The model under review builds one solid part; all positions refer to its coordinate system, in mm. A direction names the side the tool comes from. Coordinates: 2 decimals unless noted, no trailing zeros. Order: outer loops, then holes, each group sorted by start corner. A loop starts at its lowest first (then second) coordinate and runs counter-clockwise, first axis right, second up. Notation, with made-up numbers: (66.25, -37.5) - (104.25, -37.5) arc R15 cw to (104.25, -26.5) - close; hole circle Ø7 at (84.25, 2.25). An arc over 180 degrees is marked (long way). Answer in a Markdown table with one row per item.
```python
from build123d import *

# Parameters (mm, degrees)
SKETCH1_W           = 2
SKETCH1_H           = 16
BOSS_EXTRUDE1_DEPTH = 7.9375
SKETCH1_4_W         = 40
SKETCH1_4_H         = 1
BOSS_EXTRUDE2_DEPTH = 7.9375
LPATTERN1_COUNT     = 6
LPATTERN1_PITCH     = 3


with BuildPart() as part:
    # Sketch1 → Boss-Extrude1 (new body)
    with BuildSketch(Plane(origin=(0, 0, 0), x_dir=(1, 0, 0), z_dir=(0, 1, 0))):
        with Locations((-9.581037754, 12.413793103)):
            Rectangle(SKETCH1_W, SKETCH1_H)
    extrude(amount=BOSS_EXTRUDE1_DEPTH)

    # Sketch1<4> → Boss-Extrude2 (add)
    with BuildSketch(Plane(origin=(0, 0, 0), x_dir=(1, 0, 0), z_dir=(0, 1, 0))):
        with Locations((11.418962246, 19.913793103)):
            Rectangle(SKETCH1_4_W, SKETCH1_4_H)
    boss_extrude2 = extrude(amount=BOSS_EXTRUDE2_DEPTH)

    # LPattern1: Boss-Extrude2 ×6
    with Locations(*[(0, 0, i * LPATTERN1_PITCH) for i in range(1, LPATTERN1_COUNT)]):
        add(boss_extrude2)


solid = part.part
```
Item 1: Mouldability with a two-part tool opening along Z and no side actions: class faces 1 (the face through (31.419, 4, -14)), 2 (the face through (11, 4, -5.414)) as +Z half, -Z half, draft (parallel to the pull), parting line (faces both ways), or undercut.
Check values:
| item | result |
|---|---|
| face 1 | draft |
| face 2 | undercut |
Item 2: Tool access review of faces 3 (the face through (31.419, 4, -5)), 4 (the face through (-8.581, 4, -12)): name each direction out of +Z, -Z, +X, -X, +Y, -Y from which nothing blocks a thin tool from reaching the whole face with its end or side.
Check values:
| item | result |
|---|---|
| face 3 | +Z, -Z, +X, +Y, -Y |
| face 4 | +X, +Y, -Y |
Item 3: We need section C-C, the plane z = -6.25. Write out the cut boundary in (x, y), then the cut area to 3 significant figures.
Check values:
| item | result |
|---|---|
| outline | (-10.58, 0) - (-8.58, 0) - (-8.58, 7.94) - (-10.58, 7.94) - close |
| area | 15.9 mm^2 |
Item 4: We need section B-B, the plane y = 6.25. Write out the cut boundary in (x, z).
Check values:
| item | result |
|---|---|
| outline | (-10.58, -20.41) - (31.42, -20.41) - (31.42, -19.41) - (-8.58, -19.41) - (-8.58, -17.41) - (31.42, -17.41) - (31.42, -16.41) - (-8.58, -16.41) - (-8.58, -14.41) - (31.42, -14.41) - (31.42, -13.41) - (-8.58, -13.41) - (-8.58, -11.41) - (31.42, -11.41) - (31.42, -10.41) - (-8.58, -10.41) - (-8.58, -8.41) - (31.42, -8.41) - (31.42, -7.41) - (-8.58, -7.41) - (-8.58, -5.41) - (31.42, -5.41) - (31.42, -4.41) - (-10.58, -4.41) - close |
Item 5: We need section A-A, the plane x = 4. Write out the cut boundary in (y, z), then the cut area to 3 significant figures.
Check values:
| item | result |
|---|---|
| outline | (0, -20.41) - (7.94, -20.41) - (7.94, -19.41) - (0, -19.41) - close; (0, -17.41) - (7.94, -17.41) - (7.94, -16.41) - (0, -16.41) - close; (0, -14.41) - (7.94, -14.41) - (7.94, -13.41) - (0, -13.41) - close; (0, -11.41) - (7.94, -11.41) - (7.94, -10.41) - (0, -10.41) - close; (0, -8.41) - (7.94, -8.41) - (7.94, -7.41) - (0, -7.41) - close; (0, -5.41) - (7.94, -5.41) - (7.94, -4.41) - (0, -4.41) - close |
| area | 47.6 mm^2 |
Item 6: To check wall thickness, follow line 1 (Z direction, x = 3, y = 5.25); line 2 (X direction, y = 2, z = -12.5). State the ranges of each line that lie inside material, in increasing order. Write a range as from..to.
Check values:
| item | result |
|---|---|
| line 1 | -20.41..-19.41, -17.41..-16.41, -14.41..-13.41, -11.41..-10.41, -8.41..-7.41, -5.41..-4.41 |
| line 2 | -10.58..-8.58 |
Item 7: Clearance check with flat-ended pins moving along their axes: pin 1 Ø4 at (x, z) = (-3, -18.5) entering from +Y; pin 2 Ø0.6 at (y, z) = (4.5, -9.5) entering from +X; pin 3 Ø1.5 at (x, z) = (14, -6.5) entering from +Y. State where each tip first meets the part, or that it passes through.
Check values:
| item | result |
|---|---|
| pin 1 | y = 7.94 |
| pin 2 | x = -8.58 |
| pin 3 | through |
